Design review of the part built by this model. Coordinates are the model's own, in mm. A direction names the side the tool comes from. Coordinates: 2 decimals unless noted, no trailing zeros. Loops run counter-clockwise (first coordinate to the right, second up) from the corner with the lowest first, then second, coordinate; pieces in that order, holes last. Notation, with made-up numbers: M -22.5,13.25 L 0.5,13.25 A8 cw 0.5,25.25 Z; hole C 66,87 d8. An arc over 180 degrees is marked long. One line per item, written item: value.
```python
from build123d import *

# Parameters (mm, degrees)
F0_W     = 0.8
F0_H     = 12
F0_H_2   = 8
F1_DEPTH = 20


with BuildPart() as f1:
    # F0 (on Top) → F1 (new body)
    with BuildSketch(Plane.XY):
        with Locations((-2.40001, 7)):
            Rectangle(F0_W, F0_H)
        Polygon((-2.79999, -1), (2.80001, -1), (2.79999, 1), (1.99999, 1), (-2.00001, 1), (-2.80001, 1), align=None)
        with Locations((2.39999, 5)):
            Rectangle(F0_W, F0_H_2)
    extrude(amount=F1_DEPTH)


solid = f1.part
```
(1) Tool access review of faces 1 (the flat face through (0, 1, 10)), 2 (the flat face through (0, -1, 10)): name each direction out of +Z, -Z, +X, -X, +Y, -Y from which nothing blocks a thin tool from reaching the whole face with its end or side.
Reply:
face 1: +Z, -Z, +Y
face 2: +Z, -Z, +X, -X, -Y
(2) We need section D-D on y = 11.25. State the section outline as (x, z) points.
Reply:
outline: M -2.8,0 L -2,0 L -2,20 L -2.8,20 Z
(3) We need section C-C on x = -1.45. State the section outline as (y, z) points, then the cut area to 3 significant figures.
Reply:
outline: M -1,0 L 1,0 L 1,20 L -1,20 Z
area: 40.0 mm2
(4) Insertion check: pin 1 (1 mm diameter, centred on x = 0, z = 15.5, fed in from +Y). The pin has a flat end and moves straight along its axis. Give the tip position at first contact, or say it passes through.
Reply:
pin 1: stops at y = 1
(5) We need section A-A on y = 8.25. State the section outline as (x, z) points, then the cut area to 3 significant figures.
Reply:
outline: M -2.8,0 L -2,0 L -2,20 L -2.8,20 Z; M 2,0 L 2.8,0 L 2.8,20 L 2,20 Z
area: 32.0 mm2
(6) We need section B-B on z = 14. State the section outline as (x, y) points.
Reply:
outline: M -2.8,-1 L 2.8,-1 L 2.8,1 L 2.8,9 L 2,9 L 2,1 L -2,1 L -2,13 L -2.8,13 L -2.8,1 Z
(7) Mouldability with a two-part tool opening along Z and no side actions: class faces 3 (the flat face through (-2.3, 2.9, 20)), 4 (the flat face through (-2.3, 2.9, 0)), 5 (the flat face through (-2, 7, 10)) as released by +Z, released by -Z, zero draft, split by the parting line, or undercut.
Reply:
face 3: released by +Z
face 4: released by -Z
face 5: zero draft
(8) To check wall thickness, follow line 1 along X through (y, z) = (2.25, 15.5); line 2 along X through (y, z) = (11.75, 4.5); line 3 along Y through (x, z) = (-1.15, 6). State the ranges of each line that lie inside material, in increasing order. Write a range as [from, to].
Reply:
line 1: x = [-2.8, -2], [2, 2.8]
line 2: x = [-2.8, -2]
line 3: y = [-1, 1]
